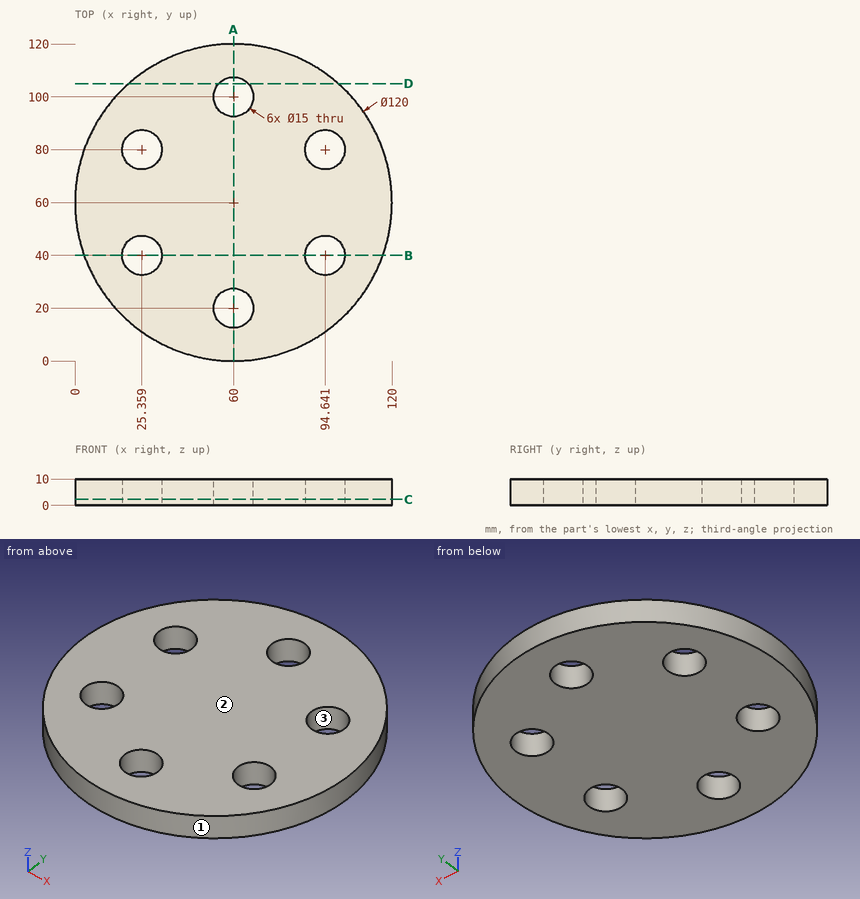
The figure shows three views and two pictorial views of one solid part (mm, origin at its lowest corner). Answer the questions. Give positions to 0.01 mm unless a question says otherwise; leave off trailing zeros. Write each loop counter-clockwise with the first axis right and the second up, starting at its lowest first coordinate (ties: lowest second). Pieces come first, ordered by that corner, then holes. Notation, with made-up numbers: (48.5, 38.25) -> (70.5, 38.25) arc R10 cw to (70.5, 53.25) -> close; hole circle Ø5 at (84.5, -5). An arc over 180 degrees is marked (long way). Write each question's results on one line, items separated by ' | '.
1. Find section B-B on y = 40. Determine the outline of the cut face in (x, z).
Data:
outline: (3.43, 0) -> (17.86, 0) -> (17.86, 10) -> (3.43, 10) -> close; (32.86, 0) -> (87.14, 0) -> (87.14, 10) -> (32.86, 10) -> close; (102.14, 0) -> (116.57, 0) -> (116.57, 10) -> (102.14, 10) -> close
2. Find section A-A on x = 60. Determine the outline of the cut face in (y, z), and give its area (3 significant figures).
Data:
outline: (0, 0) -> (12.5, 0) -> (12.5, 10) -> (0, 10) -> close; (27.5, 0) -> (92.5, 0) -> (92.5, 10) -> (27.5, 10) -> close; (107.5, 0) -> (120, 0) -> (120, 10) -> (107.5, 10) -> close | area: 900 mm^2
3. Determine the mould class of the marked faces 1, 2 and 3 for opening direction X: +X half, -X half, draft (parallel to the pull), parting line (faces both ways), or undercut.
Data:
face 1: parting line | face 2: draft | face 3: undercut
4. Find section C-C on z = 2.25. Determine the outline of the cut face in (x, y), and give its area (3 significant figures).
Data:
outline: circle Ø120 at (60, 60); hole circle Ø15 at (25.36, 40); hole circle Ø15 at (25.36, 80); hole circle Ø15 at (60, 20); hole circle Ø15 at (60, 100); hole circle Ø15 at (94.64, 40); hole circle Ø15 at (94.64, 80) | area: 10,200 mm^2
5. Each of these flat-tipped pins is pushed along its axis until it touches: pin 1 Ø5 at (y, z) = (91.5, 5.5) entering from -X; pin 2 Ø5 at (y, z) = (39, 6.5) entering from -X; pin 3 Ø6 at (y, z) = (14, 8.5) entering from -X (3 decimals); pin 4 Ø19.5 at (x, y) = (25.36, 40) entering from +Z. Where does it stop, or does it pass through?
Data:
pin 1: x = 7.47 | pin 2: x = 2.92 | pin 3: x = 18.155 | pin 4: z = 10
6. Straight lines are drawn through the part: L1, parallel to Y at x = 60, z = 3.75; L2, parallel to Y at x = 66, z = 1.75; L3, parallel to X at y = 34, z = 5.25. For each, find the intervals that lie inside material, in ascending order.
Data:
L1: 0 to 12.5, 27.5 to 92.5, 107.5 to 120 | L2: 0.3 to 15.5, 24.5 to 95.5, 104.5 to 119.7 | L3: 5.93 to 20.86, 29.86 to 90.14, 99.14 to 114.07
7. Find section D-D on y = 105. Determine the outline of the cut face in (x, z).
Data:
outline: (20.31, 0) -> (54.41, 0) -> (54.41, 10) -> (20.31, 10) -> close; (65.59, 0) -> (99.69, 0) -> (99.69, 10) -> (65.59, 10) -> close
